Build history of the part. All positions in model axes, mm. Give positions to 0.01 mm unless a question says otherwise; leave off trailing zeros. Write each loop counter-clockwise with the first axis right and the second up, starting at its lowest first coordinate (ties: lowest second). Pieces come first, ordered by that corner, then holes. Notation, with made-up numbers: (2.5, -8) -> (48.5, -8) arc R28 ccw to (48.5, 31) -> close; hole circle Ø3 at (-39, -11). An arc over 180 degrees is marked (long way). Put each result on its own line as item: value. Start each with the question number.
Item 1: Slice it at A-A, the plane z = -22. List the corners of the cut face in (x, y), plus the area to 3 significant figures.
Item 2: Slice it at C-C, the plane y = 2.1. List the corners of the cut face in (x, z), plus the area to 3 significant figures.
Item 3: Flat gauge pin, fed straight in: pin 1 Ø1.5 at (x, y) = (16, 1) entering from +Z. Where does the tip first touch, or does it go through?
Item 4: Slice it at B-B, the plane x = 13. List the corners of the cut face in (y, z), plus the area to 3 significant figures.
Item 5: Drill centre lines: line 1 along X through (y, z) = (0.2, 1); line 2 along X through (y, z) = (0.8, -22); line 3 along Z through (x, y) = (-19, 2). Where is each one in solid material? Low to high.
Item 6: Slice it at D-D, the plane z = 5.5. List the corners of the cut face in (x, y).
```python
from build123d import *

# Parameters (mm, degrees)
SKETCH_1_R      = 8.3
EXTRUDE_1_DEPTH = 3


with BuildPart() as part:
    # 草图1 → 凸台-拉伸1 (new body)
    with BuildSketch(Plane(origin=(0, 0, 0), x_dir=(1, 0, 0), z_dir=(0, 1, 0))):
        with BuildLine():
            Line((-15, 0), (-15, -10))
            Line((-15, -10), (15, -10))
            Line((15, -10), (15, 0))
            Line((15, 0), (18.2, 0))
            Line((18.2, 0), (18.2, -10))
            Line((18.2, -10), (20.7, -10))
            ThreePointArc((20.7, -10), (22.467766953, -9.267766953), (23.2, -7.5))
            Line((23.2, -7.5), (23.2, 12))
            Line((23.2, 12), (23.2, 27))
            ThreePointArc((23.2, 27), (21.735533906, 30.535533906), (18.2, 32))
            Line((18.2, 32), (-18.2, 32))
            ThreePointArc((-18.2, 32), (-21.735533906, 30.535533906), (-23.2, 27))
            Line((-23.2, 27), (-23.2, 12))
            Line((-23.2, 12), (-23.2, -7.5))
            ThreePointArc((-23.2, -7.5), (-22.467766953, -9.267766953), (-20.7, -10))
            Line((-20.7, -10), (-18.2, -10))
            Line((-18.2, -10), (-18.2, 0))
            Line((-18.2, 0), (-15, 0))
        make_face()
        with Locations(Location((13, 22, 0), (0, 0, 270))):
            Circle(SKETCH_1_R, mode=Mode.SUBTRACT)
        with Locations(Location((-13, 22, 0), (0, 0, 90))):
            Circle(SKETCH_1_R, mode=Mode.SUBTRACT)
    extrude(amount=EXTRUDE_1_DEPTH)


solid = part.part
```
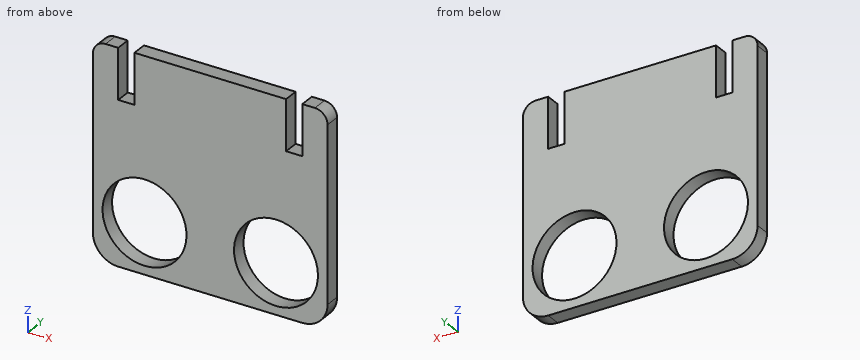
Values follow:
1. outline: (-23.2, 0) -> (-21.3, 0) -> (-21.3, 3) -> (-23.2, 3) -> close; (-4.7, 0) -> (4.7, 0) -> (4.7, 3) -> (-4.7, 3) -> close; (21.3, 0) -> (23.2, 0) -> (23.2, 3) -> (21.3, 3) -> close
1. area: 39.6 mm2
2. outline: (-23.2, -27) arc R5 ccw to (-18.2, -32) -> (18.2, -32) arc R5 ccw to (23.2, -27) -> (23.2, 7.5) arc R2.5 ccw to (20.7, 10) -> (18.2, 10) -> (18.2, 0) -> (15, 0) -> (15, 10) -> (-15, 10) -> (-15, 0) -> (-18.2, 0) -> (-18.2, 10) -> (-20.7, 10) arc R2.5 ccw to (-23.2, 7.5) -> close; hole circle Ø16.6 at (-13, -22); hole circle Ø16.6 at (13, -22)
2. area: 1,440 mm2
3. pin 1: z = 0
4. outline: (0, -32) -> (3, -32) -> (3, -30.3) -> (0, -30.3) -> close; (0, -13.7) -> (3, -13.7) -> (3, 10) -> (0, 10) -> close
4. area: 76.2 mm2
5. line 1: -23.2 to -18.2, -15 to 15, 18.2 to 23.2
5. line 2: -23.2 to -21.3, -4.7 to 4.7, 21.3 to 23.2
5. line 3: -31.94 to -27.73, -16.27 to 10
6. outline: (-23.2, 0) -> (-18.2, 0) -> (-18.2, 3) -> (-23.2, 3) -> close; (-15, 0) -> (15, 0) -> (15, 3) -> (-15, 3) -> close; (18.2, 0) -> (23.2, 0) -> (23.2, 3) -> (18.2, 3) -> close
